Could you check a few things on this drawing? It's one solid part, dimensions in mm from its lowest x, y, z. A direction names the side the tool comes from. Give positions to 0.01 mm unless a question says otherwise; leave off trailing zeros. Write each loop counter-clockwise with the first axis right and the second up, starting at its lowest first coordinate (ties: lowest second). Pieces come first, ordered by that corner, then holes. Notation, with made-up numbers: (64.5, 80) -> (113.5, 80) arc R12 cw to (113.5, 99) -> close; hole circle Ø4 at (-7.75, 84). An arc over 180 degrees is marked (long way). Use CSV: the item, a comma, the result in double quotes. Start each with the question number.
(1) Suppose I cut it at D-D on z = 26.5. List the corners of the cut face in (x, y) for me, plus the area to 3 significant figures.
(2) If we mould it in two halves opening along Y, with no side actions, what happens to the marked faces 1, 2 and 3? For each: pulls with the +Y half, pulls with the -Y half, needs draft (parallel to the pull), parting line crosses it, or undercut.
(3) Suppose I cut it at A-A on x = 40. List the corners of the cut face in (y, z) for me, plus the area to 3 significant figures.
(4) I need wall thicknesses on L1, parallel to Y at x = 40, z = 4; L2, parallel to Y at x = 71, z = 10; L3, parallel to Z at x = 53, y = 16. Which ranges of each line are inside material? Lowest first, please. Write a range as [from, to].
(5) For pin 1 Ø6 at (x, z) = (48, 35) entering from -Y; pin 2 Ø8 at (x, z) = (65, 21.5) entering from +Y; pin 3 Ø3 at (y, z) = (20, 5.5) entering from +X, each with a flat end and sliding along its axis, tell me the tip position at first contact or that it passes through.
(6) Suppose I cut it at B-B on z = 8. List the corners of the cut face in (x, y) for me, plus the area to 3 significant figures.
(7) Which directions (+Z, -Z, +X, -X, +Y, -Y) give clear straight access to the entire face, cutting with the end or side of a thin tool? Please do the marked faces 4, 5 and 6.
(8) Suppose I cut it at C-C on y = 37. List the corners of the cut face in (x, z) for me (3 decimals), plus the area to 3 significant figures.
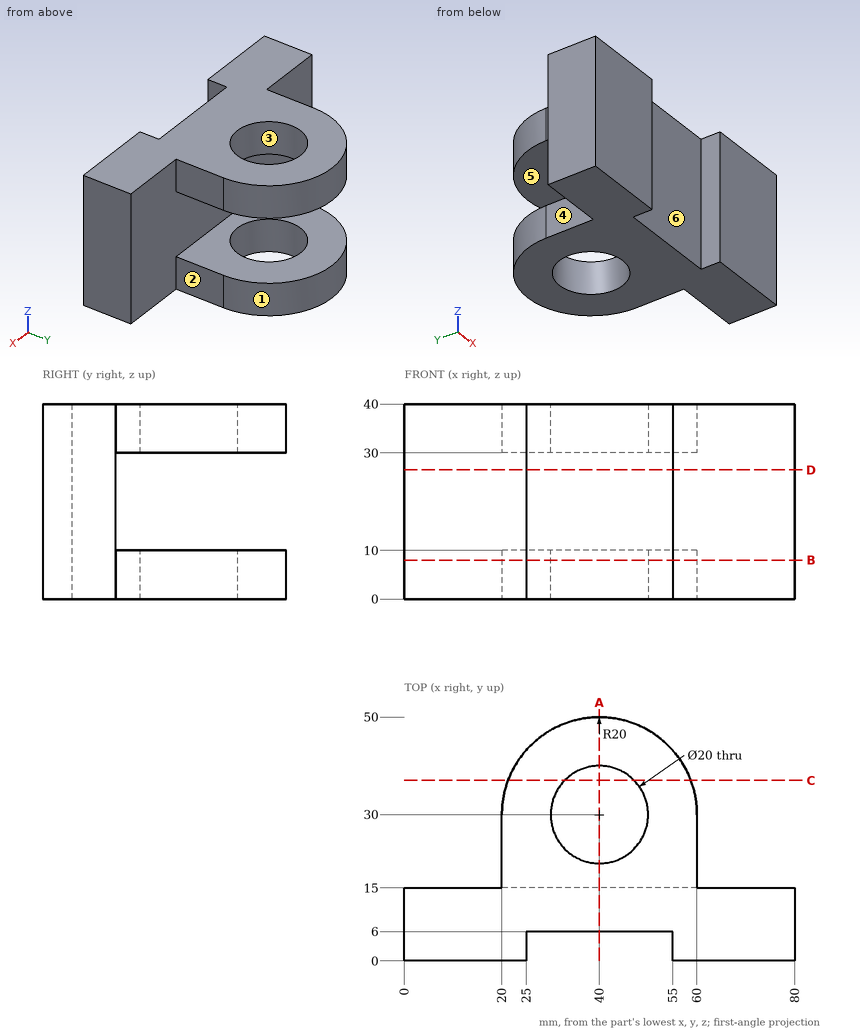
Geometry says:
1,outline,"(0, 0) -> (25, 0) -> (25, 6) -> (55, 6) -> (55, 0) -> (80, 0) -> (80, 15) -> (0, 15) -> close"
1,area,"1,020 mm²"
2,face 1,"pulls with the +Y half"
2,face 2,"needs draft"
2,face 3,"undercut"
3,outline,"(6, 0) -> (20, 0) -> (20, 10) -> (15, 10) -> (15, 30) -> (20, 30) -> (20, 40) -> (6, 40) -> close; (40, 0) -> (50, 0) -> (50, 10) -> (40, 10) -> close; (40, 30) -> (50, 30) -> (50, 40) -> (40, 40) -> close"
3,area,"660 mm²"
4,L1,"[6, 20], [40, 50]"
4,L2,"[0, 15]"
4,L3,"[0, 10], [30, 40]"
5,pin 1,"y = 6"
5,pin 2,"y = 15"
5,pin 3,"x = 60"
6,outline,"(0, 0) -> (25, 0) -> (25, 6) -> (55, 6) -> (55, 0) -> (80, 0) -> (80, 15) -> (60, 15) -> (60, 30) arc R20 ccw to (20, 30) -> (20, 15) -> (0, 15) -> close; hole circle Ø20 at (40, 30)"
6,area,"1,930 mm²"
7,face 4,"+Z, -Z, -X, +Y"
7,face 5,"+X, -X, +Y"
7,face 6,"+Z, -Z, -Y"
8,outline,"(21.265, 0) -> (32.859, 0) -> (32.859, 10) -> (21.265, 10) -> close; (21.265, 30) -> (32.859, 30) -> (32.859, 40) -> (21.265, 40) -> close; (47.141, 0) -> (58.735, 0) -> (58.735, 10) -> (47.141, 10) -> close; (47.141, 30) -> (58.735, 30) -> (58.735, 40) -> (47.141, 40) -> close"
8,area,"464 mm²"
